from build123d import *

# Parameters (mm, degrees)
EXTRUDE_1_DEPTH     = 84
CUT_EXTRUDE_1_DEPTH = 10
SKETCH_4_R          = 3
CUT_EXTRUDE_2_DEPTH = 10
SKETCH_5_W          = 22.5
SKETCH_5_H          = 21
CUT_EXTRUDE_3_DEPTH = 10


with BuildPart() as part:
    # Эскиз2 → Вытянуть-Тонкостенный1 (new body)
    with BuildSketch(Plane.XY):
        Polygon((0, 23), (0, 0), (40, 0), (40, 2), (2, 2), (2, 23), align=None)
    extrude(amount=EXTRUDE_1_DEPTH)

    # Эскиз3 → Вырез-Вытянуть1 (cut)
    with BuildSketch(Plane(origin=(0, 2, 0), x_dir=(1, 0, 0), z_dir=(0, 1, 0))):
        with BuildLine():
            Line((32, -40), (10, -40))
            ThreePointArc((10, -40), (8, -42), (10, -44))
            Line((10, -44), (32, -44))
            ThreePointArc((32, -44), (34, -42), (32, -40))
        make_face()
        with BuildLine():
            Line((18, -5), (18, -22))
            ThreePointArc((18, -22), (20, -24), (22, -22))
            Line((22, -22), (22, -5))
            ThreePointArc((22, -5), (20, -3), (18, -5))
        make_face()
        with BuildLine():
            Line((22, -79), (22, -62))
            ThreePointArc((22, -62), (20, -60), (18, -62))
            Line((18, -62), (18, -79))
            ThreePointArc((18, -79), (20, -81), (22, -79))
        make_face()
    extrude(amount=-CUT_EXTRUDE_1_DEPTH, mode=Mode.SUBTRACT)

    # Эскиз4 → Вырез-Вытянуть2 (cut)
    with BuildSketch(Plane.ZY):
        with Locations((42, 16)):
            Circle(SKETCH_4_R)
    extrude(amount=-CUT_EXTRUDE_2_DEPTH, mode=Mode.SUBTRACT)

    # Эскиз5 → Вырез-Вытянуть3 (cut)
    with BuildSketch(Plane.ZY):
        with Locations((11.25, 12.5)):
            Rectangle(SKETCH_5_W, SKETCH_5_H)
        with Locations((72.75, 12.5)):
            Rectangle(SKETCH_5_W, SKETCH_5_H)
    extrude(amount=-CUT_EXTRUDE_3_DEPTH, mode=Mode.SUBTRACT)


solid = part.part
Read the model definition and answer for the solid it produces. Units are mm, in the model's axes. A direction names the side the tool comes from. Give positions to 0.01 mm unless a question says otherwise; leave off trailing zeros. Write each loop counter-clockwise with the first axis right and the second up, starting at its lowest first coordinate (ties: lowest second). Pieces come first, ordered by that corner, then holes. Notation, with made-up numbers: (25, 9.5) - (69, 9.5) arc R28 cw to (69, 31.5) - close; hole circle Ø11 at (-37, 26). An arc over 180 degrees is marked (long way). Answer in a Markdown table with one row per item. Add a question column.
Item 1: Section A-A, the plane x = 14 is taken. Write down the section's boundary in (y, z).
Item 2: A tool of negligible diameter and unlimited length cuts with its end or side. For faces 1 (the face through (18, 1, 70)), 2 (the face through (1, 12, 61.5)), 3 (the face through (2, 12, 42)), from which of +Z, -Z, +X, -X, +Y, -Y can it reach the whole face along a straight path? Write none if from no direction.
Item 3: Determine the mould class of faces 4 (the face through (0, 12, 41)), 5 (the face through (20, 1, 0)), 6 (the face through (20, 1, 3)) for opening direction X: pulls with the +X half, pulls with the -X half, needs draft (parallel to the pull), parting line crosses it, or undercut.
Item 4: Section D-D, the plane y = 3.75 is taken. Write down the section's boundary in (x, z).
Item 5: Flat-ended cylindrical pins translate along their axes: P1, Ø5, axis at y = 13.5, z = 59, coming from the +X side; P2, Ø0.6, axis at x = 1, y = 14, coming from the +Z side; P3, Ø1.6, axis at x = 1.5, y = 10.5, coming from the -Z side. Find the tip coordinate at first contact, or state that the pin passes through.
Item 6: Section C-C, the plane z = 42 is taken. Write down the section's boundary in (x, y), and give its area (3 significant figures).
Item 7: Find the intervals of material crossed by L1, parallel to Y at x = 1.5, z = 42; L2, parallel to Y at x = 6.5, z = 36.5, in increasing order.
Item 8: Section B-B, the plane z = 69.5 is taken. Write down the section's boundary in (x, y), and give its area (3 significant figures).
Recorded:
| question | item | result |
|---|---|---|
| 1 | outline | (0, 0) - (2, 0) - (2, 40) - (0, 40) - close; (0, 44) - (2, 44) - (2, 84) - (0, 84) - close |
| 2 | face 1 | +Y, -Y |
| 2 | face 2 | +Z, +X, -X, +Y |
| 2 | face 3 | +Z, -Z, +X, +Y |
| 3 | face 4 | pulls with the -X half |
| 3 | face 5 | needs draft |
| 3 | face 6 | undercut |
| 4 | outline | (0, 22.5) - (2, 22.5) - (2, 61.5) - (0, 61.5) - close |
| 5 | P1 | stops at x = 2 |
| 5 | P2 | stops at z = 61.5 |
| 5 | P3 | stops at z = 22.5 |
| 6 | outline | (0, 0) - (8, 0) - (8, 2) - (2, 2) - (2, 13) - (0, 13) - close; (0, 19) - (2, 19) - (2, 23) - (0, 23) - close; (34, 0) - (40, 0) - (40, 2) - (34, 2) - close |
| 6 | area | 58.0 mm2 |
| 7 | L1 | y = 0 to 13, 19 to 23 |
| 7 | L2 | y = 0 to 2 |
| 8 | outline | (0, 0) - (18, 0) - (18, 2) - (0, 2) - close; (22, 0) - (40, 0) - (40, 2) - (22, 2) - close |
| 8 | area | 72.0 mm2 |
